Geometry: final body of the model. Coordinates: model frame, mm. Face numbers are marked on the shaded views. A direction names the side the tool comes from. Coordinates: 2 decimals unless noted, no trailing zeros. Order: outer loops, then holes, each group sorted by start corner. A loop starts at its lowest first (then second) coordinate and runs counter-clockwise, first axis right, second up. Notation, with made-up numbers: M 30,-8 L 56,-8 A30 ccw 56,30 Z; hole C 84,-2.5 d5. An arc over 180 degrees is marked long. One line per question, with ' | ' between items.
from build123d import *

# Parameters (mm, degrees)
SKETCH1_R         = 10.5
SKETCH1_R_2       = 6
EXTRUDE1_DEPTH    = 57
SKETCH2_R         = 9.5
EXTRUDE2_DEPTH    = 1
SKETCH3_R         = 9.5
EXTRUDE3_DEPTH    = 1
SKETCH4_OUTSIDE_W = 35.854
SKETCH4_OUTSIDE_H = 35.854
SKETCH4_OUTSIDE_R = 10
EXTRUDE4_DEPTH    = 1.3
SKETCH5_OUTSIDE_W = 35.854
SKETCH5_OUTSIDE_H = 35.854
SKETCH5_OUTSIDE_R = 10
EXTRUDE5_DEPTH    = 1.3


with BuildPart() as part:
    # Sketch1 → Extrude1 (new body)
    with BuildSketch(Plane(origin=(0, 0, 0), x_dir=(1, 0, 0), z_dir=(0, 1, 0))):
        Circle(SKETCH1_R)
        Circle(SKETCH1_R_2, mode=Mode.SUBTRACT)
    extrude(amount=EXTRUDE1_DEPTH)

    # Sketch2 → Extrude2 (cut)
    with BuildSketch(Plane(origin=(0, 57, 0), x_dir=(1, 0, 0), z_dir=(0, 1, 0))):
        Circle(SKETCH2_R)
    extrude(amount=-EXTRUDE2_DEPTH, mode=Mode.SUBTRACT)

    # Sketch3 → Extrude3 (cut)
    with BuildSketch(Plane.XZ):
        Circle(SKETCH3_R)
    extrude(amount=-EXTRUDE3_DEPTH, mode=Mode.SUBTRACT)

    # Sketch4 outside → Extrude4 (cut)
    with BuildSketch(Plane(origin=(0, 51.5, 0), x_dir=(1, 0, 0), z_dir=(0, 1, 0))):
        Rectangle(SKETCH4_OUTSIDE_W, SKETCH4_OUTSIDE_H)
        Circle(SKETCH4_OUTSIDE_R, mode=Mode.SUBTRACT)
    extrude(amount=-EXTRUDE4_DEPTH, mode=Mode.SUBTRACT)

    # Sketch5 outside → Extrude5 (cut)
    with BuildSketch(Plane(origin=(0, 5.5, 0), x_dir=(-1, 0, 0), z_dir=(0, -1, 0))):
        Rectangle(SKETCH5_OUTSIDE_W, SKETCH5_OUTSIDE_H)
        Circle(SKETCH5_OUTSIDE_R, mode=Mode.SUBTRACT)
    extrude(amount=-EXTRUDE5_DEPTH, mode=Mode.SUBTRACT)


solid = part.part
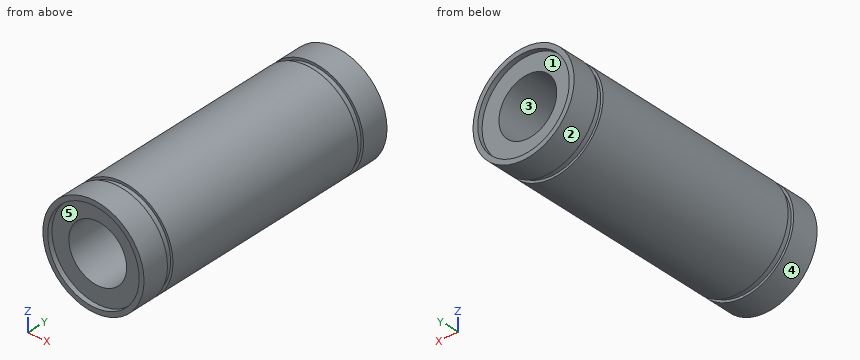
1. Access query for the marked faces 1 and 2. Directions: +Z, -Z, +X, -X, +Y, -Y. A direction counts if a zero-diameter tool reaches every point of the face in a straight line with its end or side. Return the directions, or none.
Response values:
face 1: +Y | face 2: +Y, -Y
2. Section C-C, the plane y = 13. Output: boundary loops of the cut face in (x, z), and give its area (3 significant figures).
Response values:
outline: C 0,0 d21; hole C 0,0 d12 | area: 233 mm^2
3. Material intervals for line 1 (X direction, y = 56.5, z = 0); line 2 (Z direction, x = 0, y = 42), sorted ascending. Write a range as [from, to].
Response values:
line 1: x = [-10.5, -9.5], [9.5, 10.5] | line 2: z = [-10.5, -6], [6, 10.5]
4. Draft query along Z for the marked faces 3, 4 and 5. Return one class per face: pulls with the +Z half, pulls with the -Z half, needs draft (parallel to the pull), parting line crosses it, or undercut.
Response values:
face 3: undercut | face 4: parting line crosses it | face 5: undercut
5. Section D-D, the plane z = 8.5. Output: boundary loops of the cut face in (x, y).
Response values:
outline: M -6.16,0 L -4.24,0 L -4.24,1 L 4.24,1 L 4.24,0 L 6.16,0 L 6.16,5.5 L 5.27,5.5 L 5.27,6.8 L 6.16,6.8 L 6.16,50.2 L 5.27,50.2 L 5.27,51.5 L 6.16,51.5 L 6.16,57 L 4.24,57 L 4.24,56 L -4.24,56 L -4.24,57 L -6.16,57 L -6.16,51.5 L -5.27,51.5 L -5.27,50.2 L -6.16,50.2 L -6.16,6.8 L -5.27,6.8 L -5.27,5.5 L -6.16,5.5 Z
6. Pin query (flat end, axial travel): P1, Ø6, axis at y = 48, z = -5, coming from the -X side; P2, Ø9.5, axis at x = -3, z = -3, coming from the -Y side; P3, Ø8, axis at x = -7.5, y = 49, coming from the -Z side; P4, Ø2, axis at x = -2, z = -2.5, coming from the -Y side. Return the tip coordinate at first contact, or that it passes through.
Response values:
P1: stops at x = -10.31 | P2: stops at y = 1 | P3: stops at z = -9.9 | P4: passes through
